Design review of the part built by this model. Coordinates are the model's own, in mm. A direction names the side the tool comes from. Give positions to 0.01 mm unless a question says otherwise; leave off trailing zeros. Order: outer loops, then holes, each group sorted by start corner. A loop starts at its lowest first (then second) coordinate and runs counter-clockwise, first axis right, second up. Notation, with made-up numbers: (78, 2.25) - (110, 2.25) arc R13 ccw to (110, 25.25) - close; hole circle Ø2 at (82.25, -39). An arc over 180 degrees is marked (long way). Write each question's results on one line, items separated by ' | '. Start each with the question number.
```python
from build123d import *

# Parameters (mm, degrees)
SKETCH1_W                = 11.43
SKETCH1_H                = 11.43
BOSS_EXTRUDE1_DEPTH      = 4.7625
BOSS_EXTRUDE1_DEPTH_BACK = 1.5875
SKETCH2_W                = 12.954
SKETCH2_H                = 12.954
BOSS_EXTRUDE2_DEPTH      = 1.5875
SKETCH23_W               = 4.099999912
SKETCH23_H               = 3.500000096
CUT_EXTRUDE5_DEPTH       = 8.9375
SKETCH24_W               = 6.254
SKETCH24_H               = 4.754
CUT_EXTRUDE6_DEPTH       = 4.15
SKETCH25_W               = 9.43
SKETCH25_H               = 9.43
CUT_EXTRUDE7_DEPTH       = 4.056
SKETCH26_W               = 8
SKETCH26_H               = 8
CUT_EXTRUDE8_DEPTH       = 8.9375
FILLET7_R                = 0.508
CUT_EXTRUDE9_DEPTH       = 0.38


with BuildPart() as part:
    # Sketch1 → Boss-Extrude1 (new body, two sides)
    with BuildSketch(Plane.XY) as boss_extrude1_sk:
        Rectangle(SKETCH1_W, SKETCH1_H)
    extrude(amount=BOSS_EXTRUDE1_DEPTH)
    extrude(boss_extrude1_sk.sketch, amount=-BOSS_EXTRUDE1_DEPTH_BACK)

    # Sketch2 → Boss-Extrude2 (add)
    with BuildSketch(Plane(origin=(0, 0, -1.5875), x_dir=(-1, 0, 0), z_dir=(0, 0, -1))):
        Rectangle(SKETCH2_W, SKETCH2_H)
    extrude(amount=BOSS_EXTRUDE2_DEPTH)

    # Sketch23 → Cut-Extrude5 (cut, through all)
    with BuildSketch(Plane.XY.offset(4.7625)):
        Rectangle(SKETCH23_W, SKETCH23_H)
    extrude(amount=-CUT_EXTRUDE5_DEPTH, mode=Mode.SUBTRACT)

    # Sketch24 → Cut-Extrude6 (cut)
    with BuildSketch(Plane(origin=(0, 0, -3.175), x_dir=(-1, 0, 0), z_dir=(0, 0, -1))):
        Rectangle(SKETCH24_W, SKETCH24_H)
    extrude(amount=-CUT_EXTRUDE6_DEPTH, mode=Mode.SUBTRACT)

    # Sketch25 → Cut-Extrude7 (cut)
    with BuildSketch(Plane.XY.offset(4.7625)):
        Rectangle(SKETCH25_W, SKETCH25_H)
    extrude(amount=-CUT_EXTRUDE7_DEPTH, mode=Mode.SUBTRACT)

    # Sketch26 → Cut-Extrude8 (cut, through all)
    with BuildSketch(Plane(origin=(0, 0, -3.175), x_dir=(-1, 0, 0), z_dir=(0, 0, -1))):
        Rectangle(SKETCH26_W, SKETCH26_H)
    extrude(amount=-CUT_EXTRUDE8_DEPTH, mode=Mode.SUBTRACT)

    # Fillet7
    fillet7_edges = [part.edges().sort_by_distance(p)[0] for p in [
        (4, -4, -1.23425),
        (4, 4, -1.23425),
        (-4, 4, -1.23425),
        (-4, -4, -1.23425),
        (-6.477, 6.477, -2.38125),
        (6.477, 6.477, -2.38125),
        (6.477, -6.477, -2.38125),
        (-6.477, -6.477, -2.38125),
        (5.715, -5.715, 1.5875),
        (-5.715, -5.715, 1.5875),
        (-5.715, 5.715, 1.5875),
        (5.715, 5.715, 1.5875),
        (4.715, 4.715, 2.7345),
        (4.715, -4.715, 2.7345),
        (-4.715, -4.715, 2.7345),
        (-4.715, 4.715, 2.7345),
    ]]
    fillet(fillet7_edges, radius=FILLET7_R)

    # Sketch27 → Cut-Extrude9 (cut)
    with BuildSketch(Plane.XY.offset(4.7625)):
        with BuildLine():
            Line((-5.715, 5.207), (-5.715, -5.207))
            ThreePointArc((-5.715, -5.207), (-5.566210245, -5.566210245), (-5.207, -5.715))
            Line((-5.207, -5.715), (5.207, -5.715))
            ThreePointArc((5.207, -5.715), (5.566210245, -5.566210245), (5.715, -5.207))
            Line((5.715, -5.207), (5.715, 5.207))
            ThreePointArc((5.715, 5.207), (5.566210245, 5.566210245), (5.207, 5.715))
            Line((5.207, 5.715), (-5.207, 5.715))
            ThreePointArc((-5.207, 5.715), (-5.566210245, 5.566210245), (-5.715, 5.207))
        make_face()
    extrude(amount=-CUT_EXTRUDE9_DEPTH, mode=Mode.SUBTRACT)


solid = part.part
```
Q1. For line 1 (X direction, y = 2.75, z = 0.5) (3 decimals); line 2 (X direction, y = -1, z = -2); line 3 (Y direction, x = -2, z = 3.25) (3 decimals), list the stretches that pass through material, from the lowest coordinate up. Write a range as [from, to].
Q2. Draft analysis for pull direction X (two halves, no side actions). For faces 4 (the flat face through (5.715, 0, 1)), 5 (the flat face through (-4, 0, -1)), 6 (the flat face through (0, -5.715, 1)), 7 (the flat face through (-4.3, 0.1, 0.707)), state which applies: pulls with the +X half, pulls with the -X half, needs draft (parallel to the pull), parting line crosses it, or undercut.
Q3. Add section C-C (z = 2.5). Give the boundary of the cut face in (x, y) (3 decimals).
Q4. Add section D-D (y = 5.5). Give the boundary of the cut face in (x, z) (1 decimal), plus the area to 3 significant figures.
Q5. Machinability: for faces 1 (the flat face through (-5.715, 0, 1)), 2 (the flat face through (0, 4, -1)), 3 (the flat face through (0, 4.715, 3)), which of the approach directions +Z, -Z, +X, -X, +Y, -Y give a long, thin tool a straight path to every point of the face, cutting with its end or side? Answer none if there is none.
Q6. Add section A-A (x = -1.5). Give the boundary of the cut face in (y, z) (1 decimal), plus the area to 3 significant figures.
Q7. Insertion check: pin 1 Ø4.5 at (y, z) = (1.5, -1.5) entering from -X; pin 2 Ø4 at (y, z) = (0.5, 3.5) entering from +X (3 decimals); pin 3 Ø4 at (y, z) = (1.5, 2) entering from -X (3 decimals); pin 4 Ø1.8 at (x, z) = (-1.5, 2) entering from +Y (3 decimals). Each pin has a flat end and moves straight along its axis. Give the tip position at first contact, or say it passes through.
Verdict:
1) line 1: x = [-5.715, -4], [4, 5.715] | line 2: x = [-6.48, -4], [4, 6.48] | line 3: y = [-5.715, -4.715], [4.715, 5.715]
2) face 4: pulls with the +X half | face 5: undercut | face 6: needs draft | face 7: undercut
3) outline: (-5.715, -5.207) arc R0.508 ccw to (-5.207, -5.715) - (5.207, -5.715) arc R0.508 ccw to (5.715, -5.207) - (5.715, 5.207) arc R0.508 ccw to (5.207, 5.715) - (-5.207, 5.715) arc R0.508 ccw to (-5.715, 5.207) - close; hole (-4.715, -4.207) arc R0.508 ccw to (-4.207, -4.715) - (4.207, -4.715) arc R0.508 ccw to (4.715, -4.207) - (4.715, 4.207) arc R0.508 ccw to (4.207, 4.715) - (-4.207, 4.715) arc R0.508 ccw to (-4.715, 4.207) - close
4) outline: (-6.5, -3.2) - (6.5, -3.2) - (6.5, -1.6) - (5.6, -1.6) - (5.6, 4.4) - (-5.6, 4.4) - (-5.6, -1.6) - (-6.5, -1.6) - close | area: 87.7 mm2
5) face 1: +Z, -X, +Y, -Y | face 2: +Z, -Z | face 3: +Z
6) outline: (-6.5, -3.2) - (-4, -3.2) - (-4, 0.7) - (-4.7, 0.7) - (-4.7, 4.4) - (-5.7, 4.4) - (-5.7, -1.6) - (-6.5, -1.6) - close; (4, -3.2) - (6.5, -3.2) - (6.5, -1.6) - (5.7, -1.6) - (5.7, 4.4) - (4.7, 4.4) - (4.7, 0.7) - (4, 0.7) - close | area: 23.1 mm2
7) pin 1: stops at x = -6.48 | pin 2: stops at x = 5.715 | pin 3: stops at x = -5.715 | pin 4: stops at y = 5.715
